For this review, take the finished solid that the model builds, in its own axes (mm). A direction names the side the tool comes from. Coordinates: 2 decimals unless noted, no trailing zeros. Loops run counter-clockwise (first coordinate to the right, second up) from the corner with the lowest first, then second, coordinate; pieces in that order, holes last. Notation, with made-up numbers: M 62,70 L 101,70 A15 ccw 101,95 Z; hole C 71.5,14 d10. An arc over 180 degrees is marked long. Put each result on its own line as item: value.
```python
from build123d import *

# Parameters (mm, degrees)
F0_W      = 55
F0_H      = 60
F1_DEPTH  = 12
F2_DEPTH  = 3
F3_W      = 35
F3_H      = 2
F4_DEPTH  = 56.75
F5_R      = 1.99999
F6_R      = 2
F7_DEPTH  = 63.75
F8_W      = 28
F8_H      = 3
F9_DEPTH  = 57.25
F10_SIZE  = 2
F9_FACE_W = 55
F9_FACE_H = 14
F11_DEPTH = 15
F11_TAPER = 15
F12_R     = 5


# Not quite as in the source:
# - a fillet or chamfer is up to 0.001 mm smaller than in the source, because OpenCascade refuses the exact size


with BuildPart() as f1:
    # F0 (on Top) → F1 (new body)
    with BuildSketch(Plane.XY):
        Rectangle(F0_W, F0_H)
        with BuildLine():
            ThreePointArc((-23.5, 22.25), (-24.3838834765, 24.3838834765), (-22.25, 23.5))
            Line((-22.25, 23.5), (22.25, 23.5))
            ThreePointArc((22.25, 23.5), (23.5, 24.75), (24.75, 23.5))
            ThreePointArc((24.75, 23.5), (24.3838834765, 22.6161165235), (23.5, 22.25))
            Line((23.5, 22.25), (23.5, -22.25))
            ThreePointArc((23.5, -22.25), (24.3838834765, -22.6161165235), (24.75, -23.5))
            ThreePointArc((24.75, -23.5), (23.5, -24.75), (22.25, -23.5))
            Line((22.25, -23.5), (-22.25, -23.5))
            ThreePointArc((-22.25, -23.5), (-24.3838834765, -24.3838834765), (-23.5, -22.25))
            Line((-23.5, -22.25), (-23.5, 22.25))
        make_face(mode=Mode.SUBTRACT)
        with BuildLine():
            Line((22.25, 23.5), (-22.25, 23.5))
            ThreePointArc((-22.25, 23.5), (-22.6161165235, 22.6161165235), (-23.5, 22.25))
            Line((-23.5, 22.25), (-23.5, -22.25))
            ThreePointArc((-23.5, -22.25), (-22.6161165235, -22.6161165235), (-22.25, -23.5))
            Line((-22.25, -23.5), (22.25, -23.5))
            ThreePointArc((22.25, -23.5), (22.6161165235, -22.6161165235), (23.5, -22.25))
            Line((23.5, -22.25), (23.5, 22.25))
            ThreePointArc((23.5, 22.25), (22.6161165235, 22.6161165235), (22.25, 23.5))
        make_face()
        with BuildLine():
            Line((-23.5, 22.25), (-23.5, 23.5))
            Line((-23.5, 23.5), (-22.25, 23.5))
            ThreePointArc((-22.25, 23.5), (-24.3838834765, 24.3838834765), (-23.5, 22.25))
        make_face()
        with BuildLine():
            Line((-22.25, 23.5), (-23.5, 23.5))
            Line((-23.5, 23.5), (-23.5, 22.25))
            ThreePointArc((-23.5, 22.25), (-22.6161165235, 22.6161165235), (-22.25, 23.5))
        make_face()
        with BuildLine():
            ThreePointArc((24.75, 23.5), (23.5, 24.75), (22.25, 23.5))
            Line((22.25, 23.5), (23.5, 23.5))
            Line((23.5, 23.5), (23.5, 22.25))
            ThreePointArc((23.5, 22.25), (24.3838834765, 22.6161165235), (24.75, 23.5))
        make_face()
        with BuildLine():
            Line((23.5, 23.5), (22.25, 23.5))
            ThreePointArc((22.25, 23.5), (22.6161165235, 22.6161165235), (23.5, 22.25))
            Line((23.5, 22.25), (23.5, 23.5))
        make_face()
        with BuildLine():
            ThreePointArc((24.75, -23.5), (24.3838834765, -22.6161165235), (23.5, -22.25))
            Line((23.5, -22.25), (23.5, -23.5))
            Line((23.5, -23.5), (22.25, -23.5))
            ThreePointArc((22.25, -23.5), (23.5, -24.75), (24.75, -23.5))
        make_face()
        with BuildLine():
            Line((23.5, -23.5), (23.5, -22.25))
            ThreePointArc((23.5, -22.25), (22.6161165235, -22.6161165235), (22.25, -23.5))
            Line((22.25, -23.5), (23.5, -23.5))
        make_face()
        with BuildLine():
            Line((-23.5, -23.5), (-23.5, -22.25))
            ThreePointArc((-23.5, -22.25), (-24.3838834765, -24.3838834765), (-22.25, -23.5))
            Line((-22.25, -23.5), (-23.5, -23.5))
        make_face()
        with BuildLine():
            ThreePointArc((-22.25, -23.5), (-22.6161165235, -22.6161165235), (-23.5, -22.25))
            Line((-23.5, -22.25), (-23.5, -23.5))
            Line((-23.5, -23.5), (-22.25, -23.5))
        make_face()
    extrude(amount=F1_DEPTH)

    # F0 (on Top) → F2 (join)
    with BuildSketch(Plane.XY):
        with BuildLine():
            Line((-23.5, 22.25), (-23.5, 23.5))
            Line((-23.5, 23.5), (-22.25, 23.5))
            ThreePointArc((-22.25, 23.5), (-24.3838834765, 24.3838834765), (-23.5, 22.25))
        make_face()
        with BuildLine():
            Line((-22.25, 23.5), (-23.5, 23.5))
            Line((-23.5, 23.5), (-23.5, 22.25))
            ThreePointArc((-23.5, 22.25), (-22.6161165235, 22.6161165235), (-22.25, 23.5))
        make_face()
        with BuildLine():
            Line((-23.5, -23.5), (-23.5, -22.25))
            ThreePointArc((-23.5, -22.25), (-24.3838834765, -24.3838834765), (-22.25, -23.5))
            Line((-22.25, -23.5), (-23.5, -23.5))
        make_face()
        with BuildLine():
            ThreePointArc((-22.25, -23.5), (-22.6161165235, -22.6161165235), (-23.5, -22.25))
            Line((-23.5, -22.25), (-23.5, -23.5))
            Line((-23.5, -23.5), (-22.25, -23.5))
        make_face()
        with BuildLine():
            ThreePointArc((24.75, -23.5), (24.3838834765, -22.6161165235), (23.5, -22.25))
            Line((23.5, -22.25), (23.5, -23.5))
            Line((23.5, -23.5), (22.25, -23.5))
            ThreePointArc((22.25, -23.5), (23.5, -24.75), (24.75, -23.5))
        make_face()
        with BuildLine():
            Line((23.5, -23.5), (23.5, -22.25))
            ThreePointArc((23.5, -22.25), (22.6161165235, -22.6161165235), (22.25, -23.5))
            Line((22.25, -23.5), (23.5, -23.5))
        make_face()
        with BuildLine():
            ThreePointArc((24.75, 23.5), (23.5, 24.75), (22.25, 23.5))
            Line((22.25, 23.5), (23.5, 23.5))
            Line((23.5, 23.5), (23.5, 22.25))
            ThreePointArc((23.5, 22.25), (24.3838834765, 22.6161165235), (24.75, 23.5))
        make_face()
        with BuildLine():
            Line((23.5, 23.5), (22.25, 23.5))
            ThreePointArc((22.25, 23.5), (22.6161165235, 22.6161165235), (23.5, 22.25))
            Line((23.5, 22.25), (23.5, 23.5))
        make_face()
    extrude(amount=-F2_DEPTH)

    # F3 (on face) → F4 (cut)
    with BuildSketch(Plane.YZ.offset(27.5)):
        with Locations((0, 1)):
            Rectangle(F3_W, F3_H)
    extrude(amount=-F4_DEPTH, mode=Mode.SUBTRACT)

    # F5 (radius 2 in the source; OpenCascade refuses exactly that, so slightly less here)
    f5_edges = [f1.edges().sort_by_distance(p)[0] for p in [
        (0, -17.5, 2),
        (0, 17.5, 2),
    ]]
    fillet(f5_edges, radius=F5_R)

    # F6 (on face) → F7 (cut)
    with BuildSketch(Plane(origin=(0, 30, 0), x_dir=(-1, 0, 0), z_dir=(0, 1, 0))):
        with Locations((-21, 6)):
            Circle(F6_R)
        with Locations((21, 6)):
            Circle(F6_R)
    extrude(amount=-F7_DEPTH, mode=Mode.SUBTRACT)

    # F8 (on face) → F9 (cut)
    with BuildSketch(Plane(origin=(-27.5, 0, 0), x_dir=(0, -1, 0), z_dir=(-1, 0, 0))):
        with Locations((0, 10.5)):
            Rectangle(F8_W, F8_H)
    extrude(amount=-F9_DEPTH, mode=Mode.SUBTRACT)

    # F10
    f10_edges = [f1.edges().sort_by_distance(p)[0] for p in [
        (0, -14, 12),
        (0, 14, 12),
    ]]
    chamfer(f10_edges, length=F10_SIZE)

    # F9_face (on face) → F11 (join)
    with BuildSketch(Plane(origin=(0, 23, 12), x_dir=(1, 0, 0), z_dir=(0, 0, 1))):
        Rectangle(F9_FACE_W, F9_FACE_H)
        with Locations((0, -46)):
            Rectangle(F9_FACE_W, F9_FACE_H)
    extrude(amount=F11_DEPTH, taper=F11_TAPER)

    # F12
    f12_edges = [f1.edges().sort_by_distance(p)[0] for p in [
        (-25.490381, 27.990381, 19.5),
        (25.490381, 27.990381, 19.5),
        (-25.490381, -27.990381, 19.5),
        (25.490381, -27.990381, 19.5),
    ]]
    fillet(f12_edges, radius=F12_R)


solid = f1.part
```
(1) For pin 1 (1 mm diameter, centred on x = 4.5, y = -12, fed in from +Z); pin 2 (12 mm diameter, centred on x = -8.5, y = 9, fed in from -Z); pin 3 (4 mm diameter, centred on x = 5.5, y = -22, fed in from -Z); pin 4 (3 mm diameter, centred on x = -21, z = 6, fed in from -Y), all flat-tipped, find the tip position at first contact; note any pin that passes through.
Determined:
pin 1: stops at z = 9
pin 2: stops at z = 2
pin 3: stops at z = 0
pin 4: passes through
(2) Add section B-B (y = 2.5). Write out the cut boundary in (x, z).
Determined:
outline: M -27.5,2 L 27.5,2 L 27.5,9 L -27.5,9 Z; hole C -21,6 d4; hole C 21,6 d4
(3) Add section A-A (z = 6). Write out the cut boundary in (x, y), plus the area to 3 significant figures.
Determined:
outline: M -27.5,-30 L -23,-30 L -23,30 L -27.5,30 Z; M -19,-30 L 19,-30 L 19,30 L -19,30 Z; M 23,-30 L 27.5,-30 L 27.5,30 L 23,30 Z
area: 2,820 mm^2
(4) Wall thickness on line 1 along Z through (x, y) = (21, 11); line 2 along Z through (x, y) = (-7, 5.5); line 3 along Z through (x, y) = (20, -15): over which ranges is each line inside the solid? List them lowest first. Write a range as [from, to].
Determined:
line 1: z = [2, 4], [8, 9]
line 2: z = [2, 9]
line 3: z = [2, 4.27], [7.73, 11]
(5) Tool access review of faces 1 (the flat face through (0, 0, 2)), 2 (the flat face through (0, 0, 9)), 3 (the cylindrical face through (24.037, -26.611, 19.578)): name each direction out of +Z, -Z, +X, -X, +Y, -Y from which nothing blocks a thin tool from reaching the whole face with its end or side.
Determined:
face 1: -Z, +X, -X
face 2: +Z, +X, -X
face 3: +Z, +X, -Y
(6) Draft analysis for pull direction X (two halves, no side actions). For faces 4 (the flat face through (-25.965, 20.521, 17.728)), 5 (the flat face through (0, -23, 27)), 6 (the flat face through (0, -24, 0)), state which applies: +X half, -X half, draft (parallel to the pull), parting line (faces both ways), or undercut.
Determined:
face 4: -X half
face 5: draft
face 6: undercut
